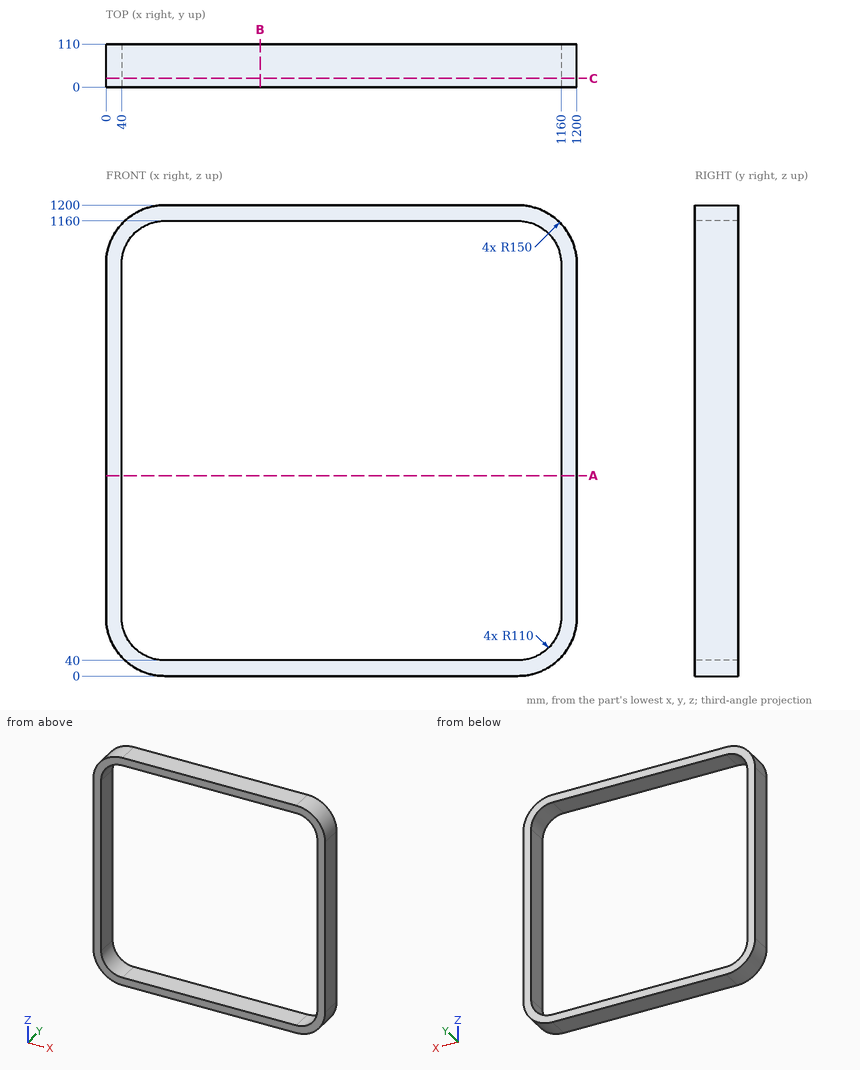
Check sheet for the drawn part. Datum: minimum x, y, z corner. Units: mm. Round coordinates to 2 decimals unless told otherwise and drop trailing zeros. Write each loop counter-clockwise with the first axis right and the second up, starting at its lowest first coordinate (ties: lowest second). Pieces come first, ordered by that corner, then holes. Notation, with made-up numbers: (21, -16) -> (59, -16) arc R12 cw to (59, 5) -> close; hole circle Ø5 at (-1.75, 42). An arc over 180 degrees is marked (long way). Put each result on its own line as item: value.
(1) Sectioned sample at C-C (y = 22.5). Enter the section's corners in (x, z).
Values found:
outline: (0, 150) arc R150 ccw to (150, 0) -> (1050, 0) arc R150 ccw to (1200, 150) -> (1200, 1050) arc R150 ccw to (1050, 1200) -> (150, 1200) arc R150 ccw to (0, 1050) -> close; hole (40, 150) arc R110 ccw to (150, 40) -> (1050, 40) arc R110 ccw to (1160, 150) -> (1160, 1050) arc R110 ccw to (1050, 1160) -> (150, 1160) arc R110 ccw to (40, 1050) -> close
(2) Sectioned sample at B-B (x = 393). Enter the section's corners in (y, z), plus the area to 3 significant figures.
Values found:
outline: (0, 0) -> (110, 0) -> (110, 40) -> (0, 40) -> close; (0, 1160) -> (110, 1160) -> (110, 1200) -> (0, 1200) -> close
area: 8,800 mm^2
(3) Sectioned sample at A-A (z = 511). Enter the section's corners in (x, y), plus the area to 3 significant figures.
Values found:
outline: (0, 0) -> (40, 0) -> (40, 110) -> (0, 110) -> close; (1160, 0) -> (1200, 0) -> (1200, 110) -> (1160, 110) -> close
area: 8,800 mm^2
(4) Material ranges on line 1 (X direction, y = 24, z = 315); line 2 (Z direction, x = 1120, y = 79) (3 decimals), recorded low to high.
Values found:
line 1: x = 0 to 40, 1160 to 1200
line 2: z = 17.335 to 65.147, 1134.853 to 1182.665
